Build history of the part. All positions in model axes, mm. Face numbers are marked on the shaded views. Round coordinates to 2 decimals unless told otherwise and drop trailing zeros. Loops run counter-clockwise (first coordinate to the right, second up) from the corner with the lowest first, then second, coordinate; pieces in that order, holes last. Notation, with made-up numbers: M 56.25,70 L 67.25,70 A6 cw 67.25,80 Z; hole C 5.25,4.25 d11. An arc over 180 degrees is marked long. One line per item, written item: value.
```python
from build123d import *

# Parameters (mm, degrees)
PIPE_TAP_DRILL_FOR_1_4_TAP1_D = 11.1252
PIPE_TAP_DRILL_FOR_1_8_TAP1_D = 8.4328
SKETCH6_R                     = 6.35
BOSS_EXTRUDE1_DEPTH           = 6.35
PIPE_TAP_DRILL_FOR_1_4_TAP2_D = 11.1252


with BuildPart() as part:
    # Sketch1 → Revolve1 (revolve)
    with BuildSketch(Plane.XY, mode=Mode.PRIVATE) as revolve1_sk:
        Polygon((0, 0), (47.498, 0), (47.498, 2.4638), (44.577, 2.4638), (44.577, 7.4422), (47.498, 7.4422), (47.498, 9.906), (41.148, 9.906), (41.148, 6.35), (0, 6.35), align=None)
    revolve(revolve1_sk.sketch.rotate(Axis((0, 48.192213231, 0), (0, -1, 0)), 180), axis=Axis((0, 48.192213231, 0), (0, -1, 0)))

    # Pipe Tap Drill for 1/4 Tap1 (through all)
    with Locations(Plane(origin=(0, 6.35, 0), x_dir=(1, 0, 0), z_dir=(0, 1, 0))):
        with Locations((0, 0), (-30.1752, 0)):
            Hole(PIPE_TAP_DRILL_FOR_1_4_TAP1_D / 2)

    # Pipe Tap Drill for 1/8 Tap1 (through all)
    with Locations(Plane(origin=(0, 6.35, 0), x_dir=(1, 0, 0), z_dir=(0, 1, 0))):
        with Locations((12.150198978, -29.333175157)):
            Hole(PIPE_TAP_DRILL_FOR_1_8_TAP1_D / 2)

    # Sketch6 → Boss-Extrude1 (add)
    with BuildSketch(Plane(origin=(0, 6.35, 0), x_dir=(1, 0, 0), z_dir=(0, 1, 0))):
        Circle(SKETCH6_R)
    extrude(amount=-BOSS_EXTRUDE1_DEPTH)

    # Pipe Tap Drill for 1/4 Tap2 (through all)
    with Locations(Plane(origin=(0, 6.35, 0), x_dir=(1, 0, 0), z_dir=(0, 1, 0))):
        with Locations((11.714341144, 10.485870911)):
            Hole(PIPE_TAP_DRILL_FOR_1_4_TAP2_D / 2)


solid = part.part
```
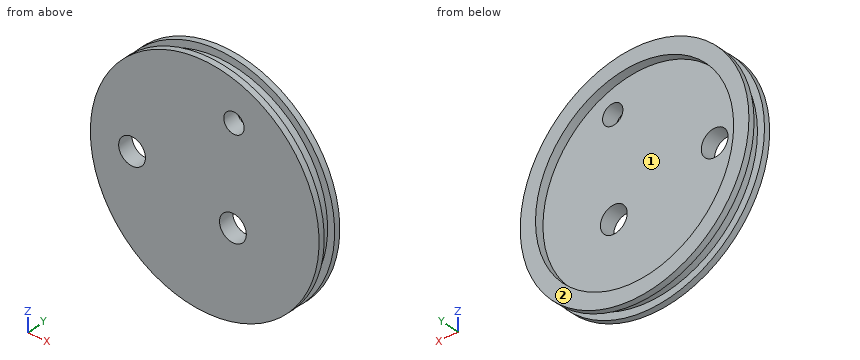
Item 1: Slice it at C-C, the plane y = 8.75. Give the cut face in (x, z), and give its area (3 significant figures).
Check values:
outline: C 0,0 d95; hole C 0,0 d82.3
area: 1,770 mm2
Item 2: Slice it at A-A, the plane z = 0. Give the cut face in (x, y).
Check values:
outline: M -47.5,0 L -35.74,0 L -35.74,6.35 L -41.15,6.35 L -41.15,9.91 L -47.5,9.91 L -47.5,7.44 L -44.58,7.44 L -44.58,2.46 L -47.5,2.46 Z; M -24.61,0 L 47.5,0 L 47.5,2.46 L 44.58,2.46 L 44.58,7.44 L 47.5,7.44 L 47.5,9.91 L 41.15,9.91 L 41.15,6.35 L -24.61,6.35 Z
Item 3: Slice it at D-D, the plane z = -22.5. Give the cut face in (x, y), and give its area (3 significant figures).
Check values:
outline: M -41.83,0 L 41.83,0 L 41.83,2.46 L 38.48,2.46 L 38.48,7.44 L 41.83,7.44 L 41.83,9.91 L 34.45,9.91 L 34.45,6.35 L -34.45,6.35 L -34.45,9.91 L -41.83,9.91 L -41.83,7.44 L -38.48,7.44 L -38.48,2.46 L -41.83,2.46 Z
area: 550 mm2
Item 4: Drop flat-ended pins along their axis: P1, Ø9, axis at x = 11.71, z = -10.49, coming from the +Y side; P2, Ø5, axis at y = 7, z = 33, coming from the -X side; P3, Ø5, axis at y = 8.5, z = 25.5, coming from the +X side; P4, Ø1, axis at y = 6, z = -22.5, coming from the -X side. Give the stop position or say it passes through.
Check values:
P1: passes through
P2: stops at x = -36.38
P3: stops at x = 41.56
P4: stops at x = -38.77
Item 5: Wall check: line 1 along Y through (x, z) = (14, -43); line 2 along Y through (x, z) = (0, 7); line 3 along X through (y, z) = (7.25, 8.5). Give the ranges that are in metal, low to high.
Check values:
line 1: y = 0 to 2.46, 7.44 to 9.91
line 2: y = 0 to 6.35
line 3: x = -43.76 to -40.26, 40.26 to 43.76
Item 6: Pull direction X, two halves, no side cores. Call the marked faces 1 and 2: pulls with the +X half, pulls with the -X half, needs draft (parallel to the pull), parting line crosses it, or undercut.
Check values:
face 1: undercut
face 2: needs draft
Item 7: Slice it at B-B, the plane x = 0. Give the cut face in (y, z).
Check values:
outline: M 0,-47.5 L 2.46,-47.5 L 2.46,-44.58 L 7.44,-44.58 L 7.44,-47.5 L 9.91,-47.5 L 9.91,-41.15 L 6.35,-41.15 L 6.35,41.15 L 9.91,41.15 L 9.91,47.5 L 7.44,47.5 L 7.44,44.58 L 2.46,44.58 L 2.46,47.5 L 0,47.5 Z
